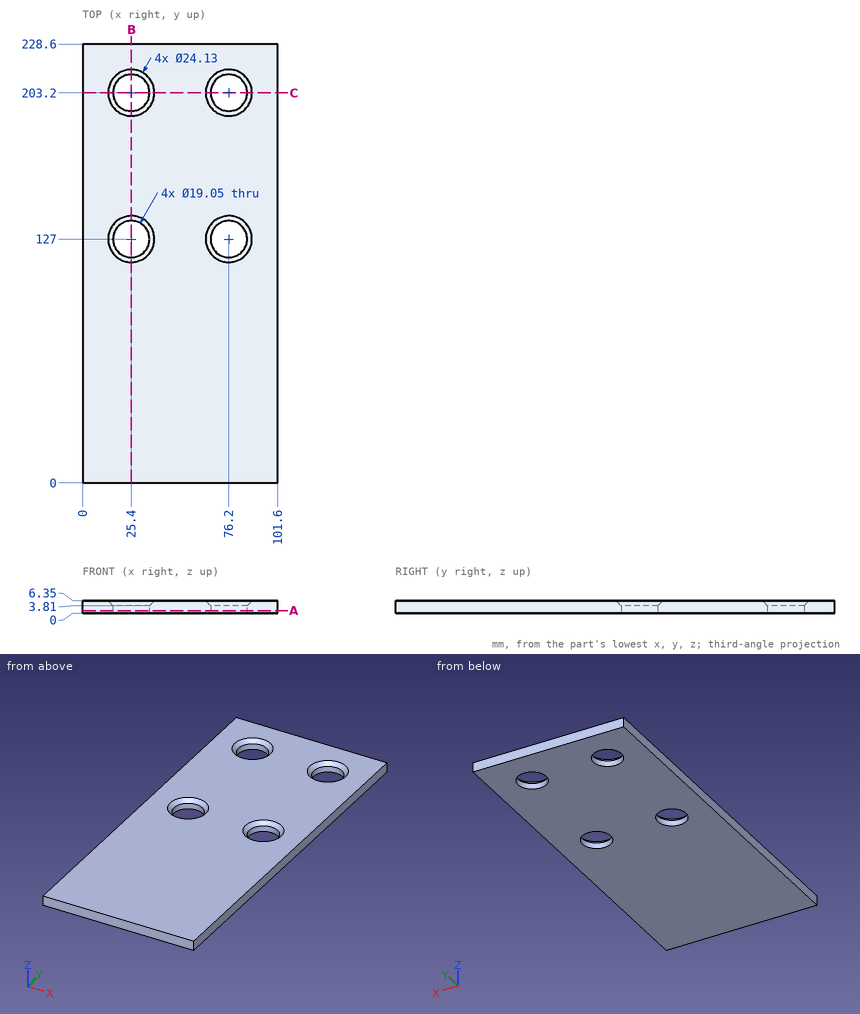
Design review of the part shown in the three views and the two pictorial views. Dimensions are in mm from the part's minimum x, y and z. Round coordinates to 2 decimals unless told otherwise and drop trailing zeros. Write each loop counter-clockwise with the first axis right and the second up, starting at its lowest first coordinate (ties: lowest second). Pieces come first, ordered by that corner, then holes. Notation, with made-up numbers: (-17, 24.5) - (-8, 24.5) arc R29 ccw to (-8, 61.5) - close; hole circle Ø11 at (29.25, 26.25). An arc over 180 degrees is marked (long way). Return JSON: item names as keys, results as strings. Group by question number.
Item 1: We need section C-C on y = 203.2. Write out the cut boundary in (x, z) (3 decimals), and give its area (3 significant figures).
Item 2: For probe 1 along Y at (x, z) = (76.2, 0.95) (3 decimals); probe 2 along X at (y, z) = (125, 4.75); probe 3 along Y at (x, z) = (18, 5), list the stretches that pass through material, from the lowest coordinate up. Write a range as [from, to].
Item 3: We need section A-A on z = 1.25. Write out the cut boundary in (x, y) (3 decimals).
Item 4: We need section B-B on x = 25.4. Write out the cut boundary in (y, z) (3 decimals).
Item 5: Insertion check: P1, Ø22, axis at x = 25.4, y = 127, coming from the +Z side (3 decimals); P2, Ø17, axis at x = 25.4, y = 203.2, coming from the -Z side. Each pin has a flat end and moves straight along its axis. Give the tip position at first contact, or say it passes through.
Model answer:
{
 "1": {"outline": "(0, 0) - (15.875, 0) - (15.875, 3.81) - (13.335, 6.35) - (0, 6.35) - close; (34.925, 0) - (66.675, 0) - (66.675, 3.81) - (64.135, 6.35) - (37.465, 6.35) - (34.925, 3.81) - close; (85.725, 0) - (101.6, 0) - (101.6, 6.35) - (88.265, 6.35) - (85.725, 3.81) - close", "area": "390 mm²"},
 "2": {"probe 1": "y = [0, 117.475], [136.525, 193.675], [212.725, 228.6]", "probe 2": "x = [0, 15.13], [35.67, 65.93], [86.47, 101.6]", "probe 3": "y = [0, 119.25], [134.75, 195.45], [210.95, 228.6]"},
 "3": {"outline": "(0, 0) - (101.6, 0) - (101.6, 228.6) - (0, 228.6) - close; hole circle Ø19.05 at (25.4, 127); hole circle Ø19.05 at (25.4, 203.2); hole circle Ø19.05 at (76.2, 127); hole circle Ø19.05 at (76.2, 203.2)"},
 "4": {"outline": "(0, 0) - (117.475, 0) - (117.475, 3.81) - (114.935, 6.35) - (0, 6.35) - close; (136.525, 0) - (193.675, 0) - (193.675, 3.81) - (191.135, 6.35) - (139.065, 6.35) - (136.525, 3.81) - close; (212.725, 0) - (228.6, 0) - (228.6, 6.35) - (215.265, 6.35) - (212.725, 3.81) - close"},
 "5": {"P1": "stops at z = 5.285", "P2": "passes through"}
}
